Build history of the part. All positions in model axes, mm. A direction names the side the tool comes from. Coordinates: 2 decimals unless noted, no trailing zeros. Order: outer loops, then holes, each group sorted by start corner. A loop starts at its lowest first (then second) coordinate and runs counter-clockwise, first axis right, second up. Notation, with made-up numbers: (62, 43) - (87, 43) arc R9 ccw to (87, 60) - close; hole circle Ø3 at (-7.75, -36). An arc over 180 degrees is marked (long way). Return JSON: item names as keys, results as strings.
Autodesk Inventor part; units mm, degrees
ref_plane "YZ Plane" through (0, 0, 0) normal (1, 0, 0) x (0, 1, 0)
ref_plane "XZ Plane" through (0, 0, 0) normal (0, 1, 0) x (-1, 0, 0)
ref_plane "XY Plane" through (0, 0, 0) normal (0, 0, 1) x (1, 0, 0)
sketch "Sketch1" plane through (0, 0, 0) normal (0, 1, 0) x (-1, 0, 0)
  line L0 (0, 0) -> (25.4, 0)
  line L1 (25.4, 0) -> (25.4, -50.8)
  line L2 (25.4, -50.8) -> (0, -50.8)
  line L3 (0, -50.8) -> (0, 0)
  line L4 (22.225, -47.625) -> (22.225, -3.175)
  line L5 (22.225, -3.175) -> (3.175, -3.175)
  line L6 (3.175, -3.175) -> (3.175, -47.625)
  line L7 (3.175, -47.625) -> (22.225, -47.625)
  dimension "d0" = 50.8
  dimension "d1" = 25.4
  dimension "d2" = 3.175
extrude "Extrusion1" add sketch "Sketch1" along normal blind 501.65
sketch "Sketch2" plane through (0, 0, 0) normal (1, 0, 0) x (0, 0, -1)
  circle A0 centre (25.4, 219.075) radius 12.7
  line L0 (0, 0) -> (0, 501.65)
  line L1 (50.8, 0) -> (0, 0)
  line L2 (50.8, 501.65) -> (0, 501.65)
  dimension "d5" = 25.4
  dimension "d6" = 25.4
  dimension "d24" = 282.575
extrude "Extrusion2" cut sketch "Sketch2" against normal blind 25.4
sketch "Sketch4" plane through (-22.225, 0, -47.625) normal (1, 0, 0) x (0, 0, -1)
  circle A0 centre (-22.225, 415.925) radius 7.62
  line L0 (-47.625, 501.65) -> (3.175, 501.65)
  line L1 (-47.625, 0) -> (-47.625, 501.65)
  dimension "d15" = 25.4
  dimension "d16" = 15.24
  dimension "d20" = 85.725
extrude "Extrusion4" cut sketch "Sketch4" against normal blind 12.7
extrude "Extrusion5" add sketch "Sketch1" against normal blind 95.25
sketch "Sketch8" plane through (-25.4, 501.65, -50.8) normal (-1, 0, 0) x (0, 0, 1)
  line L0 (47.625, -69.85) -> (3.175, -69.85)
  line L1 (3.175, -69.85) -> (3.175, -114.3)
  line L2 (3.175, -114.3) -> (47.625, -114.3)
  line L3 (47.625, -114.3) -> (47.625, -69.85)
  line L4 (0, 0) -> (50.8, 0)
  line L5 (47.625, -596.9) -> (47.625, 0)
  line L6 (3.175, 0) -> (3.175, -596.9)
  point P0 (50.8, -501.65)
  dimension "d29" = 69.85
  dimension "d30" = 0
  dimension "d31" = 0
  dimension "d32" = 44.45
extrude "Extrusion6" cut sketch "Sketch8" against normal blind 12.7 contours L3 L2 L1 L0
sketch "Sketch9" plane through (0, 501.65, 0) normal (1, 0, 0) x (0, 0, -1)
  circle A0 centre (25.4, -92.075) radius 10.16
  line L0 (0, 0) -> (50.8, 0)
  line L1 (50.8, 0) -> (50.8, -596.9)
  point P0 (0, -501.65)
  dimension "d35" = 92.075
  dimension "d36" = 25.4
  dimension "d37" = 20.32
extrude "Extrusion7" cut sketch "Sketch9" against normal blind 12.7
sketch "Sketch11" plane through (0, 501.65, -50.8) normal (0, 0, -1) x (-1, 0, 0)
  circle A0 centre (12.7, -25.4) radius 5.715
  line L0 (0, 0) -> (25.4, 0)
  line L1 (25.4, 0) -> (25.4, -596.9)
  circle A1 centre (12.7, -571.5) radius 5.715
  line L2 (25.4, -596.9) -> (0, -596.9)
  point P0 (0, -501.65)
  dimension "d48" = 11.43
  dimension "d49" = 25.4
  dimension "d50" = 12.7
  dimension "d51" = 11.43
  dimension "d52" = 12.7
  dimension "d53" = 25.4
extrude "Extrusion9" cut sketch "Sketch11" against normal blind 50.8
properties part number "2x1 16in Aluminum-ver1-1111-2020"
1. Probe L1, parallel to Y at x = -12.7, z = -1.2 (3 decimals); L2, parallel to Z at x = -12.25, y = 336 (3 decimals); L3, parallel to X at y = 140, z = -22.5 (3 decimals). List the from-to ranges inside material, lowest first.
Check values:
{"L1": "-95.25 to -75.565, -64.135 to 470.535, 481.965 to 501.65", "L2": "-50.8 to -47.625, -3.175 to 0", "L3": "-25.4 to -22.225, -3.175 to 0"}
2. Mould opens along Z. For faces 1 (the cylindrical face through (-1.565, 231.667, -23.747)), 2 (the cylindrical face through (-11.46, 470.67, -49.23)), 3 (the flat face through (-13, 207, -50.8)) say: pulls with the +Z half, pulls with the -Z half, needs draft (parallel to the pull), parting line crosses it, or undercut.
Check values:
{"face 1": "undercut", "face 2": "needs draft", "face 3": "pulls with the -Z half"}
3. Drop a flat-ended pin along its axis: pin 1 (9 mm diameter, centred on x = -12.7, y = 476.25, fed in from -Z). Give the stop position or say it passes through.
Check values:
{"pin 1": "through"}
4. Tool access for faces 4 (the flat face through (-13, 207, 0)), 5 (the flat face through (-22.225, 467, -26)): list every direction of +Z, -Z, +X, -X, +Y, -Y with a clear straight run to the whole face (end or side of a thin tool).
Check values:
{"face 4": "+Z, +X, -X, +Y, -Y", "face 5": "+Y, -Y"}
5. Cut at B-B on x = -12.7. Give the cut face in (y, z) (3 decimals), plus the area to 3 significant figures.
Check values:
{"outline": "(-95.25, -50.8) - (-75.565, -50.8) - (-75.565, -47.625) - (-95.25, -47.625) - close; (-95.25, -3.175) - (-75.565, -3.175) - (-75.565, 0) - (-95.25, 0) - close; (-64.135, -50.8) - (470.535, -50.8) - (470.535, -47.625) - (-64.135, -47.625) - close; (-64.135, -3.175) - (470.535, -3.175) - (470.535, 0) - (-64.135, 0) - close; (481.965, -50.8) - (501.65, -50.8) - (501.65, -47.625) - (481.965, -47.625) - close; (481.965, -3.175) - (501.65, -3.175) - (501.65, 0) - (481.965, 0) - close", "area": "3,650 mm²"}
6. Cut at D-D on y = 332.5. Give the cut face in (x, z) (3 decimals).
Check values:
{"outline": "(-25.4, -50.8) - (0, -50.8) - (0, 0) - (-25.4, 0) - close; hole (-22.225, -47.625) - (-3.175, -47.625) - (-3.175, -3.175) - (-22.225, -3.175) - close"}
7. Cut at C-C on y = -69.85. Give the cut face in (x, z) (3 decimals), plus the area to 3 significant figures.
Check values:
{"outline": "(-25.4, -50.8) - (-18.415, -50.8) - (-18.415, -47.625) - (-22.225, -47.625) - (-22.225, -3.175) - (-18.415, -3.175) - (-18.415, 0) - (-25.4, 0) - close; (-6.985, -50.8) - (0, -50.8) - (0, 0) - (-6.985, 0) - (-6.985, -3.175) - (-3.175, -3.175) - (-3.175, -47.625) - (-6.985, -47.625) - close", "area": "371 mm²"}
8. Cut at A-A on z = -25.4. Give the cut face in (x, y) (3 decimals).
Check values:
{"outline": "(-25.4, -95.25) - (-22.225, -95.25) - (-22.225, 206.375) - (-25.4, 206.375) - close; (-25.4, 231.775) - (-22.225, 231.775) - (-22.225, 387.35) - (-25.4, 387.35) - close; (-25.4, 431.8) - (-22.225, 431.8) - (-22.225, 501.65) - (-25.4, 501.65) - close; (-3.175, -95.25) - (0, -95.25) - (0, 206.375) - (-3.175, 206.375) - close; (-3.175, 231.775) - (0, 231.775) - (0, 399.415) - (-3.175, 399.415) - close; (-3.175, 419.735) - (0, 419.735) - (0, 501.65) - (-3.175, 501.65) - close"}
